Source: CAD feature listing. Evaluate the final solid. Frame: model axes, mm. Face numbers are marked on the shaded views. A direction names the side the tool comes from. Round coordinates to 2 decimals unless told otherwise and drop trailing zeros. Order: outer loops, then holes, each group sorted by start corner. A loop starts at its lowest first (then second) coordinate and runs counter-clockwise, first axis right, second up. Notation, with made-up numbers: (11.5, 49.25) - (39.5, 49.25) arc R18 cw to (39.5, 76.25) - close; hole circle Ø8 at (30.5, -17.75). An arc over 180 degrees is marked (long way). Return JSON: item names as keys, results as strings. Group by question number.
1) Section D-D, the plane y = -38. Return loops of the section in (x, z).
2) Ray query, line 1 (X direction, y = -15, z = -1); line 2 (Y direction, x = 3.5, z = 27.5); line 3 (Z direction, x = 6, y = -26.5). Return the intervals inside material, ascending. Write a range as from..to.
3) Access query for the marked faces 1, 2 and 3. Directions: +Z, -Z, +X, -X, +Y, -Y. A direction counts if a zero-diameter tool reaches every point of the face in a straight line with its end or side. Return the directions, or none.
4) Mould query, pull axis Y, two halves, no side actions, for the marked faces 4, 5 and 6. Classes: pulls with the +Y half, pulls with the -Y half, needs draft (parallel to the pull), parting line crosses it, or undercut.
5) Section C-C, the plane x = 22.5. Return loops of the section in (y, z).
6) Contact query for flat-ended pins moving along their axis: P1, Ø5, axis at x = 22.05, y = -15.2, coming from the +Z side; P2, Ø1.5, axis at x = 10, y = -35.5, coming from the +Z side; P3, Ø2, axis at x = 15.5, z = 4, coming from the +Y side; P4, Ø2.5, axis at y = -25.5, z = 3, coming from the +X side. Output: stop coordinate, or through.
7) Section B-B, the plane z = 47. Return loops of the section in (x, y).
8) Section A-A, the plane y = -30. Return loops of the section in (x, z).
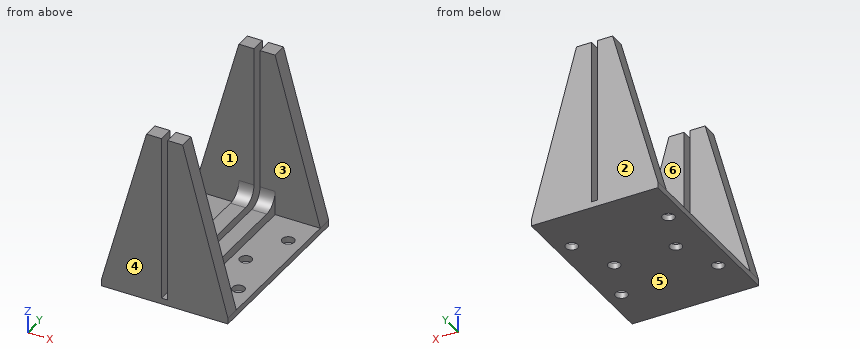
```python
from build123d import *

# Parameters (mm, degrees)
F1_DEPTH = 60
F3_DEPTH = 27.001
F4_R     = 2
F5_DEPTH = 25
F7_DEPTH = 5


with BuildPart() as f1:
    # F0 (on Front) → F1 (new body)
    with BuildSketch(Plane.XZ):
        Polygon((0, 55), (0, 0), (-15, 0), (-15, -2), (27, -2), (27, 0), (12, 0), (12, 55), (7, 55), (7, 0), (5, 0), (5, 55), align=None)
    extrude(amount=F1_DEPTH)

    # F2 (on face) → F3 (cut, through all)
    with BuildSketch(Plane(origin=(0, 0, 0), x_dir=(0, -1, 0), z_dir=(-1, 0, 0))):
        with BuildLine():
            Line((55, 55), (5, 55))
            Line((5, 55), (5, 8))
            ThreePointArc((5, 8), (6.4644660941, 4.4644660941), (10, 3))
            Line((10, 3), (50, 3))
            ThreePointArc((50, 3), (53.5355339059, 4.4644660941), (55, 8))
            Line((55, 8), (55, 55))
        make_face()
    extrude(amount=-F3_DEPTH, mode=Mode.SUBTRACT)

    # F4 (on face) → F5 (cut)
    with BuildSketch(Plane.XY):
        with Locations((-10.0474134088, -15.2)):
            Circle(F4_R)
        with Locations((-10.0474134088, -44.8)):
            Circle(F4_R)
        with Locations((-4.2247553356, -30)):
            Circle(F4_R)
        with Locations((16.2247553356, -30)):
            Circle(F4_R)
        with Locations((22.0474134088, -44.8)):
            Circle(F4_R)
        with Locations((22.0474134088, -15.2)):
            Circle(F4_R)
    extrude(amount=-F5_DEPTH, mode=Mode.SUBTRACT)



with BuildPart() as f7:
    # F6 (on face) → F7 (new body, through all)
    with BuildSketch(Plane.XZ.offset(60)):
        Polygon((0, 55), (-15, 0), (0, 0), align=None)
    extrude(amount=-F7_DEPTH)


with BuildPart() as f7b:
    # F6 (on face) → F7, piece 2 (new body, through all)
    with BuildSketch(Plane.XZ.offset(60)):
        Polygon((27, 0), (12, 55), (12, 0), align=None)
    extrude(amount=-F7_DEPTH)


with BuildPart() as f1_1:
    add(f1.part)

    add(f7.part)  # F10 merges F7

    add(f7b.part)  # F10 merges F7b
    # F10: F7b, F7 across plane
    add(f7b.part.mirror(Plane.XZ.offset(30)))
    add(f7.part.mirror(Plane.XZ.offset(30)))


solid = f1_1.part
```
Geometry check:
{
 "1": {"outline": "(-15, -2) - (27, -2) - (27, 0) - (12, 0) - (12, 3) - (7, 3) - (7, 0) - (5, 0) - (5, 3) - (0, 3) - (0, 0) - (-15, 0) - close"},
 "2": {"line 1": "-15..-12.04, -8.06..20.06, 24.04..27", "line 2": "-60..-55, -5..0", "line 3": "-2..0"},
 "3": {"face 1": "+Z, -X", "face 2": "+Z, -Z, +X, -X, +Y", "face 3": "+Z, +X"},
 "4": {"face 4": "pulls with the -Y half", "face 5": "needs draft", "face 6": "undercut"},
 "5": {"outline": "(-60, -2) - (-46.75, -2) - (-46.75, 0) - (-55, 0) - (-55, 16.5) - (-60, 16.5) - close; (-42.85, -2) - (-17.15, -2) - (-17.15, 0) - (-42.85, 0) - close; (-13.25, -2) - (0, -2) - (0, 16.5) - (-5, 16.5) - (-5, 0) - (-13.25, 0) - close"},
 "6": {"P1": "z = 0", "P2": "z = 3", "P3": "y = 0", "P4": "x = 12"},
 "7": {"outline": "(-2.18, -60) - (5, -60) - (5, -55) - (-2.18, -55) - close; (-2.18, -5) - (5, -5) - (5, 0) - (-2.18, 0) - close; (7, -60) - (14.18, -60) - (14.18, -55) - (7, -55) - close; (7, -5) - (14.18, -5) - (14.18, 0) - (7, 0) - close"},
 "8": {"outline": "(-15, -2) - (-6.22, -2) - (-6.22, 0) - (-15, 0) - close; (-2.22, -2) - (14.22, -2) - (14.22, 0) - (12, 0) - (12, 3) - (7, 3) - (7, 0) - (5, 0) - (5, 3) - (0, 3) - (0, 0) - (-2.22, 0) - close; (18.22, -2) - (27, -2) - (27, 0) - (18.22, 0) - close"}
}
